Here's how the part is built. I have some questions about the finished solid (model axes, mm). A direction names the side the tool comes from. Coordinates: 2 decimals unless noted, no trailing zeros. Write each loop counter-clockwise with the first axis right and the second up, starting at its lowest first coordinate (ties: lowest second). Pieces come first, ordered by that corner, then holes. Notation, with made-up numbers: (18.5, 50.5) -> (29.5, 50.5) arc R35 ccw to (29.5, 89.5) -> close; hole circle Ø4 at (74, -10.75). An arc over 180 degrees is marked (long way). Use a Markdown table: item, result. Add a question column.
Item 1: If we mould it in two halves opening along Z, with no side actions, what happens to faces 1 (the flat face through (0.8, 0, 2)), 2 (the flat face through (-3.185, 0, 2.5)), 3 (the cylindrical face through (1.284, -0.344, 5.029))? For each: pulls with the +Z half, pulls with the -Z half, needs draft (parallel to the pull), parting line crosses it, or undercut.
Item 2: Imagine slicing it at B-B, the plane z = -6. Write out the boundary of the cut face in (x, y), and give its area (3 significant figures).
Item 3: On a 3-axis mill with a long thin cutter (end or side, diameter ignored), from which of +Z, -Z, +X, -X, +Y, -Y can I reach the whole of each face in a straight line? I mean faces 4 (the flat face through (-3.65, -2.5, -3.8)), 5 (the flat face through (3.65, -2.5, -3.8)), 6 (the flat face through (0.645, 0, 2.5)). Say none if no direction works.
Item 4: Imagine slicing it at A-A, the plane y = -4.5. Write out the boundary of the cut face in (x, z), and give its area (3 significant figures).
Item 5: Will these pins go through, and if not, where does the flat tip stop? pin 1 Ø4 at (x, z) = (-0.5, -6) entering from +Y; pin 2 Ø1 at (x, y) = (-2.5, 1) entering from +Z; pin 3 Ø5 at (x, z) = (3.5, 4) entering from -Y; pin 4 Ø0.7 at (x, z) = (1.5, 3) entering from -Y.
Item 6: Imagine slicing it at D-D, the plane y = -1.75. Count the separate pieces of the cut face and the enclosed holes in it, and give its area (3 significant figures).
Item 7: Imagine slicing it at C-C, the plane x = 0. Write out the boundary of the cut face in (y, z).
Item 8: If I drill on line 1 along Y through (x, z) = (1.5, -5.75); line 2 along X through (y, z) = (-0.25, -0.5); line 3 along Z through (x, y) = (1, 2.5), over which ranges is the centre line in solid material (lowest first)? Write a range as from..to.
```python
from build123d import *

# Parameters (mm, degrees)
SCHIZZO1_W                   = 10.2
SCHIZZO1_H                   = 5.8
ESTRUSIONE_ESTRUSIONE1_DEPTH = 3
TAGLIO_ESTRUSIONE1_DEPTH     = 6.8
SCHIZZO3_W                   = 7.3
SCHIZZO3_H                   = 0.9
ESTRUSIONE_ESTRUSIONE2_DEPTH = 8.2
RACCORDO1_R                  = 0.5
ESTRUSIONE_ESTRUSIONE3_DEPTH = 0.32
RIPETIZIONE_A_L1_COUNT       = 3
RIPETIZIONE_A_L1_PITCH       = 2.54
RIPETIZIONE_A_L1_COL_COUNT   = 2
RIPETIZIONE_A_L1_COL_PITCH   = 2.54
SMUSSO1_SIZE                 = 0.18


with BuildPart() as part:
    # Schizzo1 → Estrusione-Estrusione1 (new body)
    with BuildSketch(Plane.XY):
        Rectangle(SCHIZZO1_W, SCHIZZO1_H)
    extrude(amount=ESTRUSIONE_ESTRUSIONE1_DEPTH)

    # Schizzo2 → Taglio-Estrusione1 (cut, through all)
    with BuildSketch(Plane(origin=(0, 2.9, 0), x_dir=(1, 0, 0), z_dir=(0, 1, 0))):
        Polygon((-4.435, -3), (-4.435, -2), (-3.185, -2), (-3.185, -3), (-1.895, -3), (-1.895, -2), (-0.645, -2), (-0.645, -3), (0.645, -3), (0.645, -2), (1.895, -2), (1.895, -3), (3.185, -3), (3.185, -2), (4.435, -2), (4.435, -3), (4.435, -3.561285121), (-4.435, -3.561285121), align=None)
    extrude(amount=-TAGLIO_ESTRUSIONE1_DEPTH, mode=Mode.SUBTRACT)

    # Schizzo3 → Estrusione-Estrusione2 (add)
    with BuildSketch(Plane(origin=(0, 0, 0), x_dir=(-1, 0, 0), z_dir=(0, 0, -1))):
        with Locations((0, -2.45)):
            Rectangle(SCHIZZO3_W, SCHIZZO3_H)
    extrude(amount=ESTRUSIONE_ESTRUSIONE2_DEPTH)

    # Raccordo1
    raccordo1_edges = [part.edges().sort_by_distance(p)[0] for p in [
        (-3.65, -2.45, -8.2),
        (3.65, -2.45, -8.2),
    ]]
    fillet(raccordo1_edges, radius=RACCORDO1_R)

    # Schizzo5 → Estrusione-Estrusione3 (add, symmetric)
    with BuildSketch(Plane(origin=(1.28, 0, 0), x_dir=(0, 0, -1), z_dir=(1, 0, 0))):
        with BuildLine():
            Line((-4.3, -0.037), (8, -0.037))
            Line((8, -0.037), (8, -0.677))
            Line((8, -0.677), (-4.3, -0.677))
            ThreePointArc((-4.3, -0.677), (-4.568700577, -0.788299423), (-4.68, -1.057))
            Line((-4.68, -1.057), (-4.68, -6.357))
            Line((-4.68, -6.357), (-5.32, -6.357))
            Line((-5.32, -6.357), (-5.32, -1.057))
            ThreePointArc((-5.32, -1.057), (-5.021248917, -0.335751083), (-4.3, -0.037))
        make_face()
    estrusione_estrusione3 = extrude(amount=ESTRUSIONE_ESTRUSIONE3_DEPTH, both=True)

    # Ripetizione a L1: Estrusione-Estrusione3 ×3
    with Locations(*[(-i * RIPETIZIONE_A_L1_PITCH, 0, 0) for i in range(1, RIPETIZIONE_A_L1_COUNT)]):
        add(estrusione_estrusione3)

    # Ripetizione a L1 col: Estrusione-Estrusione3 ×2
    with Locations(*[(i * RIPETIZIONE_A_L1_COL_PITCH, 0, 0) for i in range(1, RIPETIZIONE_A_L1_COL_COUNT)]):
        add(estrusione_estrusione3)

    # Smusso1
    smusso1_edges = [part.edges().sort_by_distance(p)[0] for p in [
        (0.96, -0.357, -8),
        (1.28, -0.677, -8),
        (1.28, -0.037, -8),
        (1.6, -0.357, -8),
        (3.5, -0.357, -8),
        (3.82, -0.677, -8),
        (3.82, -0.037, -8),
        (4.14, -0.357, -8),
        (-1.58, -0.357, -8),
        (-1.26, -0.677, -8),
        (-1.26, -0.037, -8),
        (-0.94, -0.357, -8),
        (-4.12, -0.357, -8),
        (-3.8, -0.677, -8),
        (-3.8, -0.037, -8),
        (-3.48, -0.357, -8),
    ]]
    chamfer(smusso1_edges, length=SMUSSO1_SIZE)


solid = part.part
```
Ans:
| question | item | result |
|---|---|---|
| 1 | face 1 | undercut |
| 1 | face 2 | needs draft |
| 1 | face 3 | pulls with the +Z half |
| 2 | outline | (-4.12, -0.68) -> (-3.48, -0.68) -> (-3.48, -0.04) -> (-4.12, -0.04) -> close; (-3.65, -2.9) -> (3.65, -2.9) -> (3.65, -2) -> (-3.65, -2) -> close; (-1.58, -0.68) -> (-0.94, -0.68) -> (-0.94, -0.04) -> (-1.58, -0.04) -> close; (0.96, -0.68) -> (1.6, -0.68) -> (1.6, -0.04) -> (0.96, -0.04) -> close; (3.5, -0.68) -> (4.14, -0.68) -> (4.14, -0.04) -> (3.5, -0.04) -> close |
| 2 | area | 8.21 mm^2 |
| 3 | face 4 | -Z, -X, -Y |
| 3 | face 5 | -Z, +X, -Y |
| 3 | face 6 | +Z, +Y, -Y |
| 4 | outline | (-4.12, 4.68) -> (-3.48, 4.68) -> (-3.48, 5.32) -> (-4.12, 5.32) -> close; (-1.58, 4.68) -> (-0.94, 4.68) -> (-0.94, 5.32) -> (-1.58, 5.32) -> close; (0.96, 4.68) -> (1.6, 4.68) -> (1.6, 5.32) -> (0.96, 5.32) -> close; (3.5, 4.68) -> (4.14, 4.68) -> (4.14, 5.32) -> (3.5, 5.32) -> close |
| 4 | area | 1.64 mm^2 |
| 5 | pin 1 | stops at y = -0.04 |
| 5 | pin 2 | stops at z = 3 |
| 5 | pin 3 | stops at y = -6.36 |
| 5 | pin 4 | stops at y = -0.68 |
| 6 | separate pieces | 5 |
| 6 | enclosed holes | 0 |
| 6 | area | 27.2 mm^2 |
| 7 | outline | (-2.9, -8.2) -> (-2, -8.2) -> (-2, 0) -> (2.9, 0) -> (2.9, 3) -> (-2.9, 3) -> close |
| 8 | line 1 | y = -2.9..-2, -0.68..-0.04 |
| 8 | line 2 | x = -4.12..-3.48, -1.58..-0.94, 0.96..1.6, 3.5..4.14 |
| 8 | line 3 | z = 0..2 |
